Can you work these out from the drawing? Everything is in mm from the part's minimum corner. A direction names the side the tool comes from. Give positions to 0.01 mm unless a question says otherwise; leave off trailing zeros. Loops run counter-clockwise (first coordinate to the right, second up) from the corner with the lowest first, then second, coordinate; pieces in that order, holes last.
Q1. Will these pins go through, and if not, where does the flat tip stop? P1, Ø0.6, axis at x = 5.5, z = 7, coming from the +Y side; P2, Ø1, axis at x = 14.5, z = 3, coming from the +Y side; P3, Ø4, axis at x = 13, z = 1.5, coming from the -Y side.
Q2. If we section it at B-B (y = 28): Please give me the cut outline in (x, z).
Q3. We'd pull the mould along X, two halves only. Please class the marked faces 1 and 2: +X half, -X half, draft (parallel to the pull), parting line (faces both ways), or undercut.
Q4. I need wall thicknesses on line 1 (X direction, y = 30, z = 5.5); line 2 (X direction, y = 34, z = 3.25); line 3 (Y direction, x = 16.5, z = 3). Which ranges of each line are inside material? Lowest first, please.
Q5. If we section it at C-C (x = 18.5): Please give me the cut outline in (y, z).
Q6. If we section it at A-A (z = 6): Please give me the cut outline in (x, y).
Q7. For the marked faces 3, 4 and 5, which set-ups out of +Z, -Z, +X, -X, +Y, -Y let a thin tool reach every point of the face, with its end or its side?
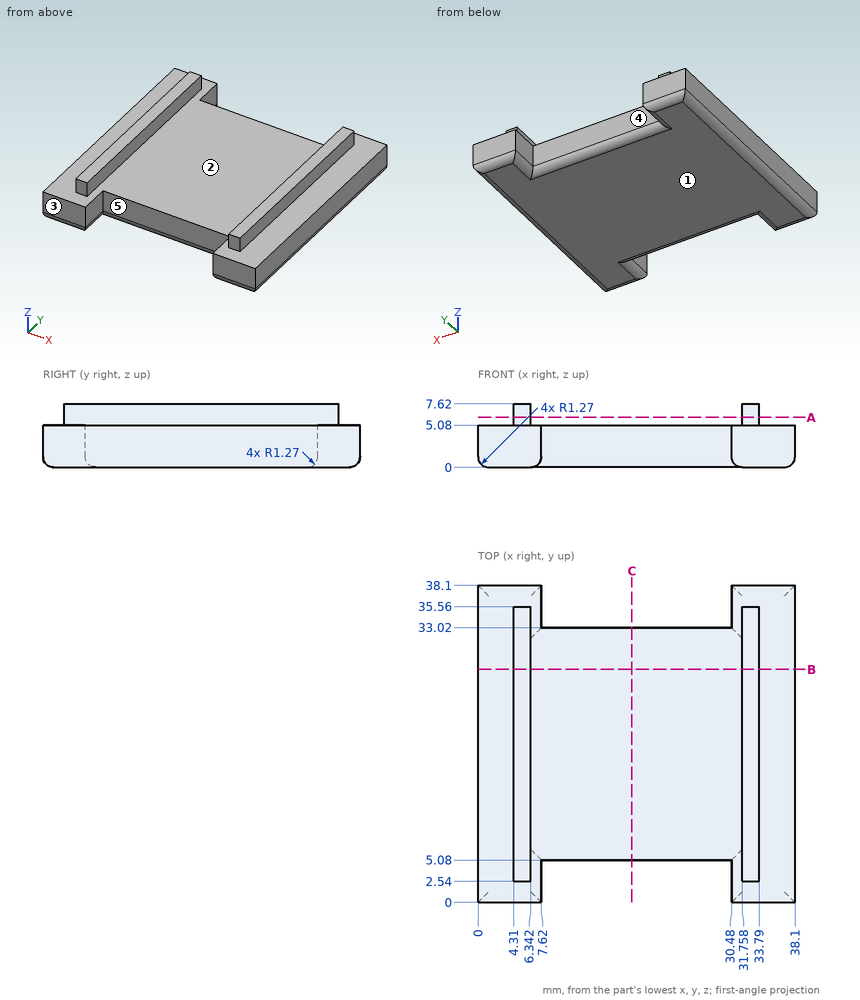
Check sheet entries:
1. P1: stops at y = 35.56
1. P2: stops at y = 33.02
1. P3: stops at y = 5.08
2. outline: (0, 1.27) arc R1.27 ccw to (1.27, 0) - (36.83, 0) arc R1.27 ccw to (38.1, 1.27) - (38.1, 5.08) - (33.79, 5.08) - (33.79, 7.62) - (31.76, 7.62) - (31.76, 5.08) - (6.34, 5.08) - (6.34, 7.62) - (4.31, 7.62) - (4.31, 5.08) - (0, 5.08) - close
3. face 1: draft
3. face 2: undercut
4. line 1: x = 4.31 to 6.34, 31.76 to 33.79
4. line 2: x = 0 to 7.62, 30.48 to 38.1
4. line 3: y = 5.08 to 33.02
5. outline: (5.08, 1.27) arc R1.27 ccw to (6.35, 0) - (31.75, 0) arc R1.27 ccw to (33.02, 1.27) - (33.02, 5.08) - (5.08, 5.08) - close
6. outline: (4.31, 2.54) - (6.34, 2.54) - (6.34, 35.56) - (4.31, 35.56) - close; (31.76, 2.54) - (33.79, 2.54) - (33.79, 35.56) - (31.76, 35.56) - close
7. face 3: +Z, -Z, +X, -X, -Y
7. face 4: +Z, -Z, +Y
7. face 5: +Z, -Z, -Y
